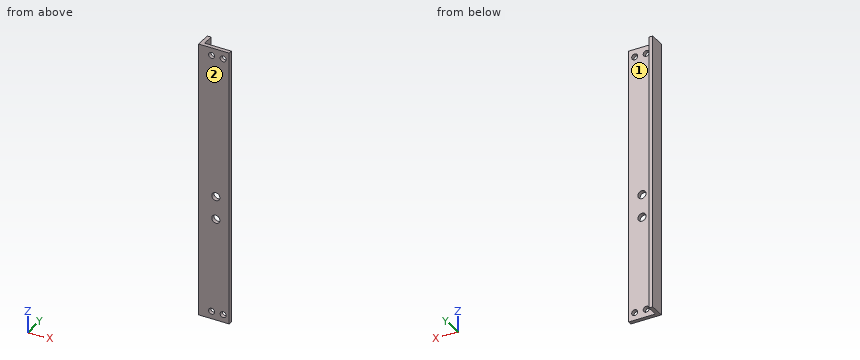
```python
from build123d import *

# Parameters (mm, degrees)
BOSS_EXTRUDE1_DEPTH = 228.6
SKETCH2_R           = 2.4892
CUT_EXTRUDE1_DEPTH  = 4.175
SKETCH3_W           = 228.6
SKETCH3_H           = 12.7
CUT_EXTRUDE2_DEPTH  = 4.175
SKETCH4_R           = 3.3655
CUT_EXTRUDE3_DEPTH  = 4.175


with BuildPart() as part:
    # Sketch1 → Boss-Extrude1 (new body)
    with BuildSketch(Plane.XY):
        Polygon((0, 0), (0, 25.4), (3.175, 25.4), (3.175, 3.175), (25.4, 3.175), (25.4, 0), align=None)
    extrude(amount=BOSS_EXTRUDE1_DEPTH)

    # Sketch2 → Cut-Extrude1 (cut, through all)
    with BuildSketch(Plane(origin=(0, 3.175, 0), x_dir=(1, 0, 0), z_dir=(0, 1, 0))):
        with Locations((20.32, -222.25)):
            Circle(SKETCH2_R)
        with Locations((10.795, -222.25)):
            Circle(SKETCH2_R)
        with Locations((20.32, -6.35)):
            Circle(SKETCH2_R)
        with Locations((10.795, -6.35)):
            Circle(SKETCH2_R)
    extrude(amount=-CUT_EXTRUDE1_DEPTH, mode=Mode.SUBTRACT)

    # Sketch3 → Cut-Extrude2 (cut, through all)
    with BuildSketch(Plane(origin=(3.175, 0, 0), x_dir=(0, 0, -1), z_dir=(1, 0, 0))):
        with Locations((-114.3, 19.05)):
            Rectangle(SKETCH3_W, SKETCH3_H)
    extrude(amount=-CUT_EXTRUDE2_DEPTH, mode=Mode.SUBTRACT)

    # Sketch4 → Cut-Extrude3 (cut, through all)
    with BuildSketch(Plane(origin=(0, 3.175, 0), x_dir=(1, 0, 0), z_dir=(0, 1, 0))):
        with Locations((14.2875, -85.09)):
            Circle(SKETCH4_R)
        with Locations((14.2875, -104.14)):
            Circle(SKETCH4_R)
    extrude(amount=-CUT_EXTRUDE3_DEPTH, mode=Mode.SUBTRACT)


solid = part.part
```
Source: CAD feature listing. Evaluate the final solid. Frame: model axes, mm. Face numbers are marked on the shaded views. A direction names the side the tool comes from. Coordinates: 2 decimals unless noted, no trailing zeros. Order: outer loops, then holes, each group sorted by start corner. A loop starts at its lowest first (then second) coordinate and runs counter-clockwise, first axis right, second up. Notation, with made-up numbers: (18.5, 3) - (76.5, 3) arc R12 cw to (76.5, 25) - close; hole circle Ø9 at (66, -16.75). An arc over 180 degrees is marked (long way). One line per item, written item: value.
1) Contact query for flat-ended pins moving along their axis: pin 1 (1 mm diameter, centred on y = 6, z = 183, fed in from +X) (3 decimals); pin 2 (9 mm diameter, centred on x = 14.29, z = 85.09, fed in from +Y) (3 decimals). Output: stop coordinate, or through.
Computed values:
pin 1: stops at x = 3.175
pin 2: stops at y = 3.175
2) Reachability of the marked faces 1 and 2 from +Z, -Z, +X, -X, +Y, -Y: full face, straight path, thin tool, end or side. Return the list, or none.
Computed values:
face 1: +Z, -Z, +X, +Y
face 2: +Z, -Z, +X, -X, -Y
3) Cut plane B-B on x = 20.32. Output: boundary loops of the cut face in (y, z) (3 decimals), plus the area to 3 significant figures.
Computed values:
outline: (0, 0) - (3.175, 0) - (3.175, 3.861) - (0, 3.861) - close; (0, 8.839) - (3.175, 8.839) - (3.175, 219.761) - (0, 219.761) - close; (0, 224.739) - (3.175, 224.739) - (3.175, 228.6) - (0, 228.6) - close
area: 694 mm^2
4) Ray query, line 1 (X direction, y = 0.95, z = 6.35); line 2 (Z direction, x = 14.5, y = 2.5); line 3 (Z direction, x = 20.32, y = 0.8). Return the intervals inside material, ascending. Write a range as [from, to].
Computed values:
line 1: x = [0, 8.31], [13.28, 17.83], [22.81, 25.4]
line 2: z = [0, 81.73], [88.45, 100.78], [107.5, 228.6]
line 3: z = [0, 3.86], [8.84, 219.76], [224.74, 228.6]
5) Cut plane D-D on z = 149.5. Output: boundary loops of the cut face in (x, y) (3 decimals), plus the area to 3 significant figures.
Computed values:
outline: (0, 0) - (25.4, 0) - (25.4, 3.175) - (3.175, 3.175) - (3.175, 12.7) - (0, 12.7) - close
area: 111 mm^2
6) Cut plane A-A on z = 6.35. Output: boundary loops of the cut face in (x, y) (3 decimals), plus the area to 3 significant figures.
Computed values:
outline: (0, 0) - (8.306, 0) - (8.306, 3.175) - (3.175, 3.175) - (3.175, 12.7) - (0, 12.7) - close; (13.284, 0) - (17.831, 0) - (17.831, 3.175) - (13.284, 3.175) - close; (22.809, 0) - (25.4, 0) - (25.4, 3.175) - (22.809, 3.175) - close
area: 79.3 mm^2
7) Cut plane C-C on z = 104.14. Output: boundary loops of the cut face in (x, y) (3 decimals), plus the area to 3 significant figures.
Computed values:
outline: (0, 0) - (10.922, 0) - (10.922, 3.175) - (3.175, 3.175) - (3.175, 12.7) - (0, 12.7) - close; (17.653, 0) - (25.4, 0) - (25.4, 3.175) - (17.653, 3.175) - close
area: 89.5 mm^2
